from build123d import *

# Parameters (mm, degrees)
SKETCH1_R           = 1.5
BOSS_EXTRUDE1_DEPTH = 4


with BuildPart() as part:
    # Sketch1 → Boss-Extrude1 (new body)
    with BuildSketch(Plane.XY):
        with BuildLine():
            Line((49.000000342, 3.999999998), (49.000000342, -2e-09))
            Line((49.000000342, -2e-09), (63.000000342, -2e-09))
            Line((63.000000342, -2e-09), (63.000000342, 3.999999998))
            Line((63.000000342, 3.999999998), (68.000000342, 3.999999998))
            Line((68.000000342, 3.999999998), (68.000000342, 26.999999998))
            ThreePointArc((68.000000342, 26.999999998), (65.071068153, 34.07106781), (58.000000342, 36.999999998))
            Line((58.000000342, 36.999999998), (10.000000342, 36.999999998))
            ThreePointArc((10.000000342, 36.999999998), (2.92893253, 34.07106781), (3.42e-07, 26.999999998))
            Line((3.42e-07, 26.999999998), (3.42e-07, 3.999999998))
            Line((3.42e-07, 3.999999998), (5.000000342, 3.999999998))
            Line((5.000000342, 3.999999998), (5.000000342, -2e-09))
            Line((5.000000342, -2e-09), (19.000000342, -2e-09))
            Line((19.000000342, -2e-09), (19.000000342, 3.999999998))
            Line((19.000000342, 3.999999998), (27.000000342, 3.999999998))
            Line((27.000000342, 3.999999998), (27.000000342, -2e-09))
            Line((27.000000342, -2e-09), (41.000000342, -2e-09))
            Line((41.000000342, -2e-09), (41.000000342, 3.999999998))
            Line((41.000000342, 3.999999998), (49.000000342, 3.999999998))
        make_face()
        with Locations((10.000000342, 14.999999998)):
            Circle(SKETCH1_R, mode=Mode.SUBTRACT)
        with Locations((10.000000342, 25.499999998)):
            Circle(SKETCH1_R, mode=Mode.SUBTRACT)
        with Locations((58.000000342, 14.999999998)):
            Circle(SKETCH1_R, mode=Mode.SUBTRACT)
        with Locations((58.000000342, 25.499999998)):
            Circle(SKETCH1_R, mode=Mode.SUBTRACT)
        with Locations((6.500000342, 30.499999998)):
            Circle(SKETCH1_R, mode=Mode.SUBTRACT)
        Polygon((54.500000342, 30.499999998), (54.500000342, 21.499999998), (58.000000342, 21.499999998), (58.000000342, 18.999999998), (54.500000342, 18.999999998), (54.500000342, 9.999999998), (13.500000342, 9.999999998), (13.500000342, 18.999999998), (10.000000342, 18.999999998), (10.000000342, 21.499999998), (13.500000342, 21.499999998), (13.500000342, 30.499999998), align=None, mode=Mode.SUBTRACT)
    extrude(amount=BOSS_EXTRUDE1_DEPTH)


solid = part.part
Here's how the part is built. I have some questions about the finished solid (model axes, mm). A direction names the side the tool comes from. Round coordinates to 2 decimals unless told otherwise and drop trailing zeros. Write each loop counter-clockwise with the first axis right and the second up, starting at its lowest first coordinate (ties: lowest second). Pieces come first, ordered by that corner, then holes.
1. Suppose I cut it at D-D (z = 2.45). State how many separate pieces and enclosed holes the cut face has, and give its area (3 significant figures).
2. Suppose I cut it at C-C (x = 48). List the corners of the cut face in (y, z) for me.
3. Will these pins go through, and if not, where does the flat tip stop? pin 1 Ø2.5 at (x, y) = (58, 25.5) entering from -Z; pin 2 Ø2 at (y, z) = (2, 1.5) entering from +X; pin 3 Ø2 at (y, z) = (1, 2.5) entering from -X; pin 4 Ø2 at (y, z) = (33, 0.5) entering from -X.
4. I need wall thicknesses on L1, parallel to X at y = 15, z = 1.6; L2, parallel to X at y = 14, z = 0.55; L3, parallel to Y at x = 35, z = 1.05. Which ranges of each line are inside material? Lowest first, please.
5. If we mould it in two halves opening along X, with no side actions, what happens to faces 5 (the cylindrical face through (65.15, 33.99, 1.97)), 6 (the flat face through (49, 2, 2)), 7 (the flat face through (34, 31, 4))? For each: released by +X, released by -X, zero draft, split by the parting line, or undercut.
6. Suppose I cut it at A-A (x = 55.5). List the corners of the cut face in (y, z) for me.
7. For faces 1 (the flat face through (12, 21.5, 2)), 2 (the flat face through (45, 4, 2)), 3 (the flat face through (65, 4, 2)), 4 (the flat face through (2, 4, 2)), which set-ups out of +Z, -Z, +X, -X, +Y, -Y let a thin tool reach every point of the face, with its end or its side?
8. Suppose I cut it at B-B (y = 25.5). List the corners of the cut face in (x, z) for me.
Answer sheet:
1. separate pieces: 1
1. enclosed holes: 6
1. area: 1,480 mm2
2. outline: (4, 0) - (10, 0) - (10, 4) - (4, 4) - close; (30.5, 0) - (37, 0) - (37, 4) - (30.5, 4) - close
3. pin 1: passes through
3. pin 2: stops at x = 63
3. pin 3: stops at x = 5
3. pin 4: stops at x = 1.34
4. L1: x = 0 to 8.5, 11.5 to 13.5, 54.5 to 56.5, 59.5 to 68
4. L2: x = 0 to 8.88, 11.12 to 13.5, 54.5 to 56.88, 59.12 to 68
4. L3: y = 0 to 10, 30.5 to 37
5. face 5: released by +X
5. face 6: undercut
5. face 7: zero draft
6. outline: (0, 0) - (19, 0) - (19, 4) - (0, 4) - close; (21.5, 0) - (37, 0) - (37, 4) - (21.5, 4) - close
7. face 1: +Z, -Z
7. face 2: +Z, -Z, -Y
7. face 3: +Z, -Z, +X, -Y
7. face 4: +Z, -Z, -X, -Y
8. outline: (0, 0) - (8.5, 0) - (8.5, 4) - (0, 4) - close; (11.5, 0) - (13.5, 0) - (13.5, 4) - (11.5, 4) - close; (54.5, 0) - (56.5, 0) - (56.5, 4) - (54.5, 4) - close; (59.5, 0) - (68, 0) - (68, 4) - (59.5, 4) - close
